Read the model definition and answer for the solid it produces. Units are mm, in the model's axes. Round coordinates to 2 decimals unless told otherwise and drop trailing zeros. Use one line per item in the form item = value. Start each with the question number.
from build123d import *

# Parameters (mm, degrees)
BOSS_EXTRU_1_DEPTH                                 = 300
CHAMBRAGE_POUR_VIS_T_TE_HEXAGONALE_M31_D           = 3.5
CHAMBRAGE_POUR_VIS_T_TE_HEXAGONALE_M31_DEPTH       = 8.000000001
CHAMBRAGE_POUR_VIS_T_TE_HEXAGONALE_M31_CBORE_D     = 6
CHAMBRAGE_POUR_VIS_T_TE_HEXAGONALE_M31_CBORE_DEPTH = 4.500000001


with BuildPart() as part:
    # Esquisse1 → Boss.-Extru.1 (new body)
    with BuildSketch(Plane(origin=(-167.5, 0, 0), x_dir=(0, -1, 0), z_dir=(-1, 0, 0))):
        with BuildLine():
            Line((-157, 193.75), (-168, 193.75))
            Line((-168, 193.75), (-168.5, 193.25))
            Line((-168.5, 193.25), (-168.5, 189.607879579))
            ThreePointArc((-168.5, 189.607879579), (-168.4576137, 189.468608075), (-168.344827586, 189.376562202))
            ThreePointArc((-168.344827586, 189.376562202), (-168.01524529, 189.174071401), (-167.767205011, 188.877249849))
            ThreePointArc((-167.767205011, 188.877249849), (-167.685241932, 188.792985122), (-167.573828324, 188.755495145))
            Line((-167.573828324, 188.755495145), (-167.228211064, 188.725257552))
            ThreePointArc((-167.228211064, 188.725257552), (-167.065680666, 188.64510643), (-167, 188.476208878))
            Line((-167, 188.476208878), (-167, 188.023787121))
            ThreePointArc((-167, 188.023787121), (-167.065680666, 187.854889569), (-167.228211064, 187.774738446))
            Line((-167.228211064, 187.774738446), (-167.59477657, 187.74266812))
            ThreePointArc((-167.59477657, 187.74266812), (-167.703244499, 187.707004425), (-167.784541491, 187.626829678))
            ThreePointArc((-167.784541491, 187.626829678), (-168.027906161, 187.347614221), (-168.344827586, 187.155915383))
            ThreePointArc((-168.344827586, 187.155915383), (-168.4576137, 187.06386951), (-168.5, 186.924598006))
            Line((-168.5, 186.924598006), (-168.5, 186.249999999))
            Line((-168.5, 186.249999999), (-168, 185.749999999))
            Line((-168, 185.749999999), (-157, 185.749999999))
            Line((-157, 185.749999999), (-156.5, 186.249999999))
            Line((-156.5, 186.249999999), (-156.5, 186.924598006))
            ThreePointArc((-156.5, 186.924598006), (-156.5423863, 187.06386951), (-156.655172414, 187.155915383))
            ThreePointArc((-156.655172414, 187.155915383), (-156.972093839, 187.347614221), (-157.215458509, 187.626829678))
            ThreePointArc((-157.215458509, 187.626829678), (-157.296755501, 187.707004425), (-157.40522343, 187.74266812))
            Line((-157.40522343, 187.74266812), (-157.771788936, 187.774738446))
            ThreePointArc((-157.771788936, 187.774738446), (-157.934319334, 187.854889569), (-158, 188.023787121))
            Line((-158, 188.023787121), (-158, 188.476208878))
            ThreePointArc((-158, 188.476208878), (-157.934319334, 188.64510643), (-157.771788936, 188.725257552))
            Line((-157.771788936, 188.725257552), (-157.426171676, 188.755495145))
            ThreePointArc((-157.426171676, 188.755495145), (-157.314758068, 188.792985122), (-157.232794989, 188.877249849))
            ThreePointArc((-157.232794989, 188.877249849), (-156.98475471, 189.174071401), (-156.655172414, 189.376562202))
            ThreePointArc((-156.655172414, 189.376562202), (-156.5423863, 189.468608075), (-156.5, 189.607879579))
            Line((-156.5, 189.607879579), (-156.5, 193.25))
            Line((-156.5, 193.25), (-157, 193.75))
        make_face()
    extrude(amount=-BOSS_EXTRU_1_DEPTH)

    # Chambrage pour vis à tête hexagonale M31
    with Locations(Plane(origin=(0, 0, 185.749999999), x_dir=(-1, 0, 0), z_dir=(0, 0, -1))):
        with Locations((155, 162.5), (130, 162.5), (105, 162.5), (80, 162.5), (55, 162.5), (30, 162.5), (5, 162.5), (-20, 162.5), (-45, 162.5), (-70, 162.5), (-95, 162.5), (-120, 162.5), (-147.5, 162.5)):
            CounterBoreHole(CHAMBRAGE_POUR_VIS_T_TE_HEXAGONALE_M31_D / 2, CHAMBRAGE_POUR_VIS_T_TE_HEXAGONALE_M31_CBORE_D / 2, CHAMBRAGE_POUR_VIS_T_TE_HEXAGONALE_M31_CBORE_DEPTH, depth=CHAMBRAGE_POUR_VIS_T_TE_HEXAGONALE_M31_DEPTH)


solid = part.part
Item 1: Given P1, Ø2, axis at x = 95, y = 162.5, coming from the -Z side; P2, Ø1.8, axis at x = -56, y = 163, coming from the -Z side, each flat-ended and moving along its own axis, determine where each tip first touches the part or whether it passes through.
Item 2: Find the intervals of material crossed by L1, parallel to Y at x = 70, z = 186.7; L2, parallel to Y at x = 45, z = 191.85; L3, parallel to Y at x = 34, z = 188, in increasing order. Write a range as [from, to].
Item 3: For a pull along Y with two mould halves and no side action, classify faces 1 (the flat face through (-167.5, 163, 190)), 2 (the flat face through (70, 160.5, 190.25)), 3 (the cylindrical face through (97.21, 164.53, 187.97)) as pulls with the +Y half, pulls with the -Y half, needs draft (parallel to the pull), parting line crosses it, or undercut.
The answers:
q1.P1 = through
q1.P2 = 190.25
q2.L1 = [156.5, 159.5], [165.5, 168.5]
q2.L2 = [156.5, 160.75], [164.25, 168.5]
q2.L3 = [158, 167]
q3.face_1 = needs draft
q3.face_2 = undercut
q3.face_3 = undercut
